Input: part model. Units: mm. Frame: model coordinates. Face numbers are marked on the shaded views. A direction names the side the tool comes from. Coordinates: 2 decimals unless noted, no trailing zeros. Loops run counter-clockwise (first coordinate to the right, second up) from the corner with the lowest first, then second, coordinate; pieces in that order, holes last. Notation, with made-up numbers: (9.25, -34.75) - (57.25, -34.75) arc R23 cw to (57.25, 0.25) - close; hole circle Ø3 at (51, -17). An arc over 180 degrees is marked (long way). Use one line per item in the form item = value.
from build123d import *

# Parameters (mm, degrees)
SKETCH2_R                   = 4.5
BOSS_EXTRUDE1_DEPTH         = 5
SKETCH3_R                   = 5.95
BOSS_EXTRUDE2_DEPTH         = 12
SKETCH4_R                   = 10
BOSS_EXTRUDE3_DEPTH         = 5
M3_TAPPED_HOLE1_D           = 2.5
M3_TAPPED_HOLE1_CSINK_D     = 3.05
M3_TAPPED_HOLE1_CSINK_ANGLE = 90
SKETCH11_W                  = 2
SKETCH11_H                  = 3
CUT_EXTRUDE2_DEPTH          = 5
SKETCH12_R                  = 4
BOSS_EXTRUDE5_DEPTH         = 35


with BuildPart() as part:
    # Sketch2 → Boss-Extrude1 (new body)
    with BuildSketch(Plane(origin=(0, 0, 0), x_dir=(1, 0, 0), z_dir=(0, 1, 0))):
        with Locations(Location((0, 0, 0), (0, 0, 270))):
            Circle(SKETCH2_R)
    extrude(amount=BOSS_EXTRUDE1_DEPTH)

    # Sketch3 → Boss-Extrude2 (add)
    with BuildSketch(Plane(origin=(0, 5, 0), x_dir=(1, 0, 0), z_dir=(0, 1, 0))):
        with Locations(Location((0, 0, 0), (0, 0, 270))):
            Circle(SKETCH3_R)
    extrude(amount=BOSS_EXTRUDE2_DEPTH)

    # Sketch4 → Boss-Extrude3 (add)
    with BuildSketch(Plane(origin=(0, 17, 0), x_dir=(1, 0, 0), z_dir=(0, 1, 0))):
        with Locations(Location((0, 0, 0), (0, 0, 270))):
            Circle(SKETCH4_R)
    extrude(amount=BOSS_EXTRUDE3_DEPTH)

    # M3 Tapped Hole1 (through all)
    with Locations(Plane(origin=(0, 0, 0), x_dir=(-1, 0, 0), z_dir=(0, -1, 0))):
        with Locations((0, 0)):
            CounterSinkHole(M3_TAPPED_HOLE1_D / 2, M3_TAPPED_HOLE1_CSINK_D / 2, counter_sink_angle=M3_TAPPED_HOLE1_CSINK_ANGLE)

    # Sketch11 → Cut-Extrude2 (cut)
    with BuildSketch(Plane.XZ):
        with Locations((0, 4.5)):
            Rectangle(SKETCH11_W, SKETCH11_H)
    extrude(amount=-CUT_EXTRUDE2_DEPTH, mode=Mode.SUBTRACT)

    # Sketch12 → Boss-Extrude5 (add)
    with BuildSketch(Plane(origin=(0, 22, 0), x_dir=(1, 0, 0), z_dir=(0, 1, 0))):
        with Locations(Location((0, 0, 0), (0, 0, 270))):
            Circle(SKETCH12_R)
    extrude(amount=BOSS_EXTRUDE5_DEPTH)


solid = part.part
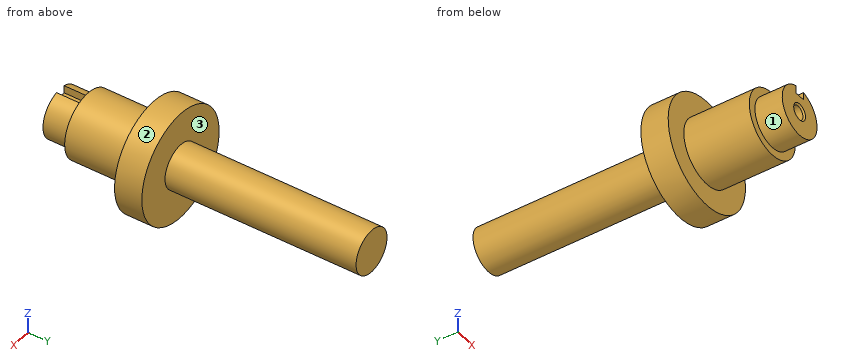
Q1. Cut plane B-B, the plane x = 0. Return loops of the section in (y, z) (3 decimals), then the cut area to 3 significant figures.
Check values:
outline = (0, -4.5) - (5, -4.5) - (5, -5.95) - (17, -5.95) - (17, -10) - (22, -10) - (22, -4) - (57, -4) - (57, 4) - (22, 4) - (22, 10) - (17, 10) - (17, 5.95) - (5, 5.95) - (5, 3) - (0, 3) - (0, 1.525) - (0.275, 1.25) - (22, 1.25) - (22, -1.25) - (0.275, -1.25) - (0, -1.525) - close
area = 505 mm²
Q2. First-contact query: P1, Ø0.7, axis at y = 1.5, z = 3.5, coming from the +X side; P2, Ø0.7, axis at y = 2, z = 3.5, coming from the -X side; P3, Ø4, axis at x = 2, y = 35, coming from the -Z side; P4, Ø3, axis at x = 7, y = 47.5, coming from the +Z side. Flat tips, straight axial feed; report the tip coordinate or a pass-through.
Check values:
P1 = 3.21
P2 = -3.21
P3 = -4
P4 = through
Q3. Cut plane D-D, the plane y = 31. Return loops of the section in (x, z).
Check values:
outline = circle Ø8 at (0, 0)
Q4. Cut plane C-C, the plane y = 9. Return loops of the section in (x, z), then the cut area to 3 significant figures.
Check values:
outline = circle Ø11.9 at (0, 0); hole circle Ø2.5 at (0, 0)
area = 106 mm²
Q5. Cut plane A-A, the plane z = 0. Return loops of the section in (x, y) (3 decimals).
Check values:
outline = (-10, 17) - (-5.95, 17) - (-5.95, 5) - (-4.5, 5) - (-4.5, 0) - (-1.525, 0) - (-1.25, 0.275) - (-1.25, 22) - (1.25, 22) - (1.25, 0.275) - (1.525, 0) - (4.5, 0) - (4.5, 5) - (5.95, 5) - (5.95, 17) - (10, 17) - (10, 22) - (4, 22) - (4, 57) - (-4, 57) - (-4, 22) - (-10, 22) - close
Q6. Set-up query: the marked faces 1, 2 and 3. Return all of +Z, -Z, +X, -X, +Y, -Y with unobstructed straight access to the full face (end or side cutting, diameter ignored); none if empty.
Check values:
face_1 = -Y
face_2 = +Y, -Y
face_3 = +Y
Q7. Ray query, line 1 along Y through (x, z) = (-8.25, 3); line 2 along Z through (x, y) = (0.75, 7); line 3 along Y through (x, z) = (-3.75, 2). Return the intervals inside material, ascending. Write a range as [from, to].
Check values:
line_1 = [17, 22]
line_2 = [-5.9, -1], [1, 5.9]
line_3 = [0, 22]
